Geometry: final body of the model. Coordinates: model frame, mm. A direction names the side the tool comes from. Give positions to 0.01 mm unless a question says otherwise; leave off trailing zeros. Write each loop counter-clockwise with the first axis right and the second up, starting at its lowest first coordinate (ties: lowest second). Pieces come first, ordered by that corner, then holes.
Q1. Draft query along X for faces 1 (the face through (1, 0, 31.65)), 2 (the face through (0.2, 0, 31)), 3 (the face through (-0.29, 2.23, 22.16)). Return one class per face: pulls with the +X half, pulls with the -X half, needs draft (parallel to the pull), parting line crosses it, or undercut.
Q2. Cut plane A-A on y = 0. Return the cut outline in (x, z).
Q3. Cut plane B-B on z = 28. Return the cut outline in (x, y).
Q4. Line query: L1, parallel to Z at x = 0.15, y = 0.7; L2, parallel to Y at x = -0.15, z = 22 (3 decimals); L3, parallel to Z at x = 1.2, y = -0.15. Output: solid intervals per line, ascending.
Q5. Pin query (flat end, axial travel): pin 1 (1.5 mm diameter, centred on y = 0, z = 23.5, fed in from +X); pin 2 (1 mm diameter, centred on y = 0.5, z = 9, fed in from +X). Return the tip coordinate at first contact, or that it passes through.
Q6. Reachability of faces 4 (the face through (-0.314, -1.416, 27.087)), 5 (the face through (-2, 0, 21.65)), 6 (the face through (-1, 0, 31.65)), 7 (the face through (-0.2, 0, 31)) from +Z, -Z, +X, -X, +Y, -Y: full face, straight path, thin tool, end or side. Return the list, or none.
Q7. Cut plane C-C on x = -1.9. Return the cut outline in (y, z), plus the area to 3 significant figures.
Q8. Cut plane D-D on z = 8. Return the cut outline in (x, y).
```python
from build123d import *

# Parameters (mm, degrees)
SKETCH_1_R          = 1.5
EXTRUDE_1_DEPTH     = 22.65
SKETCH_2_R          = 1.45
EXTRUDE_2_DEPTH     = 9
CUT_EXTRUDE_1_DEPTH = 1
SKETCH_4_R          = 1.5
SKETCH_4_R_2        = 1
CUT_EXTRUDE_2_DEPTH = 2
SKETCH_5_R          = 2.25
EXTRUDE_3_DEPTH     = 1


with BuildPart() as part:
    # 草图1 → 凸台-拉伸1 (new body)
    with BuildSketch(Plane.XY):
        Circle(SKETCH_1_R)
    extrude(amount=EXTRUDE_1_DEPTH)

    # 草图2 → 凸台-拉伸2 (add)
    with BuildSketch(Plane.XY.offset(22.65)):
        Circle(SKETCH_2_R)
    extrude(amount=EXTRUDE_2_DEPTH)

    # 草图3 → 切除-拉伸1 (cut)
    with BuildSketch(Plane.XY.offset(31.65)):
        with BuildLine():
            Line((-0.2, -1.486606875), (-0.2, 1.486606875))
            ThreePointArc((-0.2, 1.486606875), (0, 1.5), (0.2, 1.486606875))
            Line((0.2, 1.486606875), (0.2, -1.486606875))
            ThreePointArc((0.2, -1.486606875), (0, -1.5), (-0.2, -1.486606875))
        make_face()
    extrude(amount=-CUT_EXTRUDE_1_DEPTH, mode=Mode.SUBTRACT)

    # 草图4 → 切除-拉伸2 (cut)
    with BuildSketch(Plane(origin=(0, 0, 0), x_dir=(-1, 0, 0), z_dir=(0, 0, -1))):
        Circle(SKETCH_4_R)
        Circle(SKETCH_4_R_2, mode=Mode.SUBTRACT)
    extrude(amount=-CUT_EXTRUDE_2_DEPTH, mode=Mode.SUBTRACT)

    # 草图5 → 凸台-拉伸3 (add)
    with BuildSketch(Plane.XY.offset(22.65)):
        Circle(SKETCH_5_R)
    extrude(amount=-EXTRUDE_3_DEPTH)


solid = part.part
```
Data:
1. face 1: needs draft
1. face 2: undercut
1. face 3: parting line crosses it
2. outline: (-2.25, 21.65) - (-1.5, 21.65) - (-1.5, 2) - (-1, 2) - (-1, 0) - (1, 0) - (1, 2) - (1.5, 2) - (1.5, 21.65) - (2.25, 21.65) - (2.25, 22.65) - (1.45, 22.65) - (1.45, 31.65) - (0.2, 31.65) - (0.2, 30.65) - (-0.2, 30.65) - (-0.2, 31.65) - (-1.45, 31.65) - (-1.45, 22.65) - (-2.25, 22.65) - close
3. outline: circle Ø2.9 at (0, 0)
4. L1: z = 0 to 30.65
4. L2: y = -2.245 to 2.245
4. L3: z = 2 to 31.65
5. pin 1: stops at x = 1.45
5. pin 2: stops at x = 1.5
6. face 4: +Z
6. face 5: -Z
6. face 6: +Z, +X, -X, +Y, -Y
6. face 7: +Z, +Y, -Y
7. outline: (-1.21, 21.65) - (1.21, 21.65) - (1.21, 22.65) - (-1.21, 22.65) - close
7. area: 2.41 mm2
8. outline: circle Ø3 at (0, 0)
